Autodesk Inventor part; units mm, degrees
ref_plane "YZ Plane" through (0, 0, 0) normal (1, 0, 0) x (0, 1, 0)
ref_plane "XZ Plane" through (0, 0, 0) normal (0, 1, 0) x (-1, 0, 0)
ref_plane "XY Plane" through (0, 0, 0) normal (0, 0, 1) x (1, 0, 0)
sketch "Esboço1" plane through (0, 0, 0) normal (0, 1, 0) x (-1, 0, 0)
  line L0 (0, 0) -> (68, 0)
  line L1 (68, 0) -> (68, -68)
  line L2 (68, -68) -> (0, -68)
  line L3 (0, -68) -> (0, 0)
  line L4 (66, -2) -> (2, -2)
  line L5 (2, -2) -> (2, -66)
  line L6 (2, -66) -> (66, -66)
  line L7 (66, -66) -> (66, -2)
  dimension "d0" = 68
  dimension "d1" = 68
  dimension "d2" = 2
  dimension "d3" = 2
  dimension "d4" = 2
  dimension "d5" = 2
extrude "Extrusão1" add sketch "Esboço1" along normal blind 38
sketch "Esboço2" plane through (0, 38, 0) normal (0, 1, 0) x (1, 0, 0)
  line L0 (-68, 68) -> (0, 68)
  line L1 (0, 0) -> (-68, 0)
  line L2 (-68, 0) -> (-68, 68)
  line L3 (-68, 68) -> (0, 68)
  line L4 (0, 68) -> (0, 0)
extrude "Extrusão2" add sketch "Esboço2" along normal blind 2
chamfer "Chanfro1" distance 2 angle 45 8 edges at (-68, 20, -68) (0, 20, -68) (-68, 20, 0) (0, 20, 0) (0, 40, -34) (-34, 40, -68) (-68, 40, -34) (-34, 40, 0)
sketch "Esboço3" plane through (0, 0, -2) normal (1, 0, 0) x (0, 0, -1)
  line L0 (64, 0) -> (0, 0) construction
  line L1 (32, 11) -> (32, 0) construction
  line L2 (43.5, 11) -> (20.5, 11)
  line L3 (20.5, 11) -> (20.5, 7)
  line L4 (20.5, 7) -> (43.5, 7)
  line L5 (43.5, 7) -> (43.5, 11)
  point P0 (-2, 0)
  dimension "d16" = 4
  dimension "d17" = 11
  dimension "d18" = 23
extrude "Extrusão3" cut sketch "Esboço3" against normal blind 4
sketch "Esboço4" plane through (-68, 0, -66) normal (-1, 0, 0) x (0, 0, 1)
  line L0 (43.5, 11) -> (20.5, 11)
  line L1 (43.5, 7) -> (20.5, 7)
  line L2 (20.5, 7) -> (20.5, 11)
  line L3 (20.5, 11) -> (43.5, 11)
  line L4 (43.5, 11) -> (43.5, 7)
  point P0 (66, 0)
extrude "Extrusão4" cut sketch "Esboço4" against normal blind 4
sketch "Esboço5" plane through (0, 40, 0) normal (0, 1, 0) x (1, 0, 0)
  line L0 (-34, 66) -> (-34, 2) construction
  line L1 (-43, 49) -> (-47, 49)
  line L2 (-47, 49) -> (-47, 19)
  line L3 (-47, 19) -> (-43, 19)
  line L4 (-43, 19) -> (-43, 49)
  line L5 (-43, 34) -> (-61.5633, 34) construction
  line L6 (-66, 2) -> (-66, 66) construction
  arc A0 (-62.5279, 39.2371) -> (-56.6721, 39.2371) centre (-59.6, 34) ccw
  ellipse E0 centre (-59.6, 40) end of major axis (-56.6, 40) minor radius 3.5 (-56.6721, 39.2371) -> (-62.5279, 39.2371) ccw
  line L7 (-25, 49) -> (-21, 49)
  line L8 (-21, 49) -> (-21, 19)
  line L9 (-21, 19) -> (-25, 19)
  line L10 (-25, 19) -> (-25, 49)
  arc A1 (-11.3279, 39.2371) -> (-5.4721, 39.2371) centre (-8.4, 34) ccw
  ellipse E1 centre (-8.4, 40) end of major axis (-11.4, 40) minor radius 3.5 (-5.4721, 39.2371) -> (-11.3279, 39.2371) ccw
  point P0 (0, 0)
  dimension "d28" = 3
  dimension "d29" = 3.5
  dimension "d23" = 4
  dimension "d24" = 30
  dimension "d25" = 19
  dimension "d26" = 12
  dimension "d27" = 6.4
extrude "Extrusão5" cut sketch "Esboço5" against normal blind 4
sketch "Esboço6" plane through (0, 38, 0) normal (0, -1, 0) x (1, 0, 0)
  point P0 (0, 0)
sketch "Esboço7" plane through (0, 38, 0) normal (0, -1, 0) x (1, 0, 0)
  line L0 (-15, -2) -> (-17, -2)
  line L1 (-17, -2) -> (-17, -66)
  line L2 (-17, -66) -> (-15, -66)
  line L3 (-15, -66) -> (-15, -2)
  line L4 (-2, -2) -> (-2, -66)
  line L5 (-34, -66) -> (-34, -2) construction
  line L6 (-15, -2) -> (-17, -2) construction
  line L7 (-15, -2) -> (-17, -2)
  line L8 (-53, -2) -> (-51, -2)
  line L9 (-51, -2) -> (-51, -66)
  line L10 (-51, -66) -> (-53, -66)
  line L11 (-53, -66) -> (-53, -2)
  point P0 (0, 0)
  dimension "d32" = 2
  dimension "d33" = 13
extrude "Extrusão6" add sketch "Esboço7" along normal blind 14
properties part number "BundOtta"
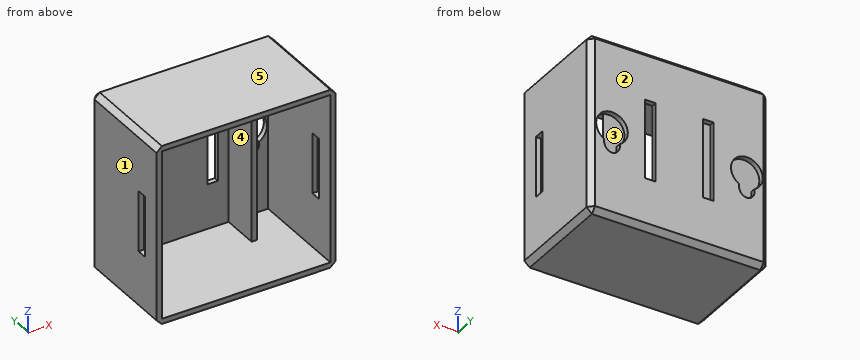
The listing builds one solid part. Answer for the finished solid, in the listing's coordinates (mm). Face numbers are marked on the shaded views. A direction names the side the tool comes from. Round coordinates to 2 decimals unless told otherwise and drop trailing zeros. Order: outer loops, then holes, each group sorted by start corner. A loop starts at its lowest first (then second) coordinate and runs counter-clockwise, first axis right, second up. Notation, with made-up numbers: (36.5, -3.5) - (67.5, -3.5) arc R35 ccw to (67.5, 30.5) - close; hole circle Ø6 at (53, 29). An arc over 180 degrees is marked (long way). Write item = value, one per line. Start each with the question number.
1) Section A-A, the plane y = 22 is taken. Write down the section's boundary in (x, z), plus the area to 3 significant figures.
2) For the marked faces 4 and 5, determine the directions among +Z, -Z, +X, -X, +Y, -Y from which every point of the face is accessible in a straight line to the end or side of a thin tool.
3) Section C-C, the plane y = 27 is taken. Write down the section's boundary in (x, z), plus the area to 3 significant figures.
4) Straight lines are drawn through the part: L1, parallel to X at y = 36, z = -31; L2, parallel to X at y = 38.7, z = -34; L3, parallel to Z at x = -54, y = 22.5. For each, find the intervals that lie inside material, in ascending order.
5) Section D-D, the plane x = -55.5 is taken. Write down the section's boundary in (y, z), plus the area to 3 significant figures.
6) Section B-B, the plane x = -19 is taken. Write down the section's boundary in (y, z), plus the area to 3 significant figures.
7) For a pull along X with two mould halves and no side action, classify the marked faces 1, 2 and 3 as released by +X, released by -X, zero draft, split by the parting line, or undercut.
8) Given pin 1 (0.6 mm diameter, centred on x = -66.5, z = -30, fed in from +Y); pin 2 (1.6 mm diameter, centred on x = -1, z = -39.5, fed in from -Y); pin 3 (10 mm diameter, centred on x = -17, z = -30, fed in from -Y); pin 4 (4 mm diameter, centred on x = -11.5, z = -42.5, fed in from -Y), each flat-ended and moving along its own axis, determine where each tip first touches the part or whether it passes through.
Results list:
q1.outline = (-68, -66) - (-66, -68) - (-2, -68) - (0, -66) - (0, -2) - (-2, 0) - (-66, 0) - (-68, -2) - close; hole (-66, -66) - (-2, -66) - (-2, -2) - (-66, -2) - close
q1.area = 520 mm^2
q2.face_4 = -Y
q2.face_5 = +Z, +X, -X, +Y, -Y
q3.outline = (-68, -66) - (-66, -68) - (-2, -68) - (0, -66) - (0, -2) - (-2, 0) - (-66, 0) - (-68, -2) - close; hole (-66, -66) - (-53, -66) - (-53, -2) - (-66, -2) - close; hole (-51, -66) - (-17, -66) - (-17, -2) - (-51, -2) - close; hole (-15, -66) - (-2, -66) - (-2, -2) - (-15, -2) - close
q3.area = 776 mm^2
q4.L1 = -68 to -66, -53 to -51, -17 to -15, -2 to 0
q4.L2 = -67.3 to -65.6, -53.6 to -47, -43 to -25, -21 to -14.4, -2.4 to -0.7
q4.L3 = -68 to -66, -2 to 0
q5.outline = (0, -68) - (38, -68) - (40, -66) - (40, -38.38) - (38, -38.38) - (38, -66) - (0, -66) - close; (0, -2) - (38, -2) - (38, -29.62) - (40, -29.62) - (40, -2) - (38, 0) - (0, 0) - close
q5.area = 266 mm^2
q6.outline = (0, -68) - (38, -68) - (40, -66) - (40, -2) - (38, 0) - (0, 0) - (0, -2) - (38, -2) - (38, -66) - (0, -66) - close
q6.area = 284 mm^2
q7.face_1 = released by -X
q7.face_2 = zero draft
q7.face_3 = undercut
q8.pin_1 = 39.8
q8.pin_2 = 0
q8.pin_3 = 24
q8.pin_4 = 38
